Geometry check sheet. Reference: the model listing, model coordinates, mm. Face numbers are marked on the shaded views. A direction names the side the tool comes from. Give positions to 0.01 mm unless a question says otherwise; leave off trailing zeros. Order: outer loops, then holes, each group sorted by start corner. A loop starts at its lowest first (then second) coordinate and runs counter-clockwise, first axis right, second up.
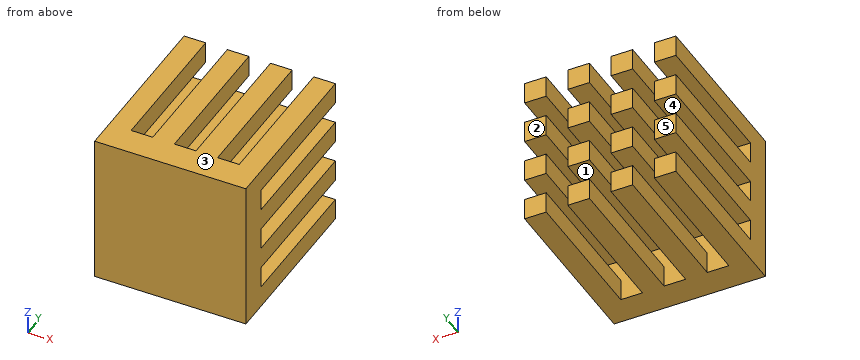
```python
from build123d import *

# Parameters (mm, degrees)
SKETCH1_W            = 10.5
SKETCH1_H            = 10.5
BOSS_EXTRUDE1_DEPTH  = 2
SKETCH2_W            = 1.5
SKETCH2_H            = 1.5
BOSS_EXTRUDE2_DEPTH  = 10
LPATTERN1_COUNT      = 4
LPATTERN1_PITCH      = 3
LPATTERN1_COUNT_DIR2 = 4
LPATTERN1_PITCH_DIR2 = 3


with BuildPart() as part:
    # Sketch1 → Boss-Extrude1 (new body)
    with BuildSketch(Plane(origin=(0, 0, 0), x_dir=(1, 0, 0), z_dir=(0, 1, 0))):
        Rectangle(SKETCH1_W, SKETCH1_H)
    extrude(amount=BOSS_EXTRUDE1_DEPTH)

    # Sketch2 → Boss-Extrude2 (add)
    with BuildSketch(Plane(origin=(0, 2, 0), x_dir=(1, 0, 0), z_dir=(0, 1, 0))):
        with Locations((-4.5, 4.5)):
            Rectangle(SKETCH2_W, SKETCH2_H)
    boss_extrude2 = extrude(amount=BOSS_EXTRUDE2_DEPTH)

    # LPattern1: Boss-Extrude2 4 × 4
    with Locations(*[(i * LPATTERN1_PITCH, 0, j * LPATTERN1_PITCH_DIR2) for i in range(LPATTERN1_COUNT) for j in range(LPATTERN1_COUNT_DIR2) if (i, j) != (0, 0)]):
        add(boss_extrude2)


solid = part.part
```
Q1. Access from +Z, -Z, +X, -X, +Y, -Y to the whole of each face (thin tool, end or side, straight path). Record for the marked faces 4 and 5.
Q2. Cross-section at B-B, the plane x = -1. Record the boundary of the cut face in (y, z).
Q3. Gauge pin test, flat end, axial feed: P1, Ø1, axis at x = 0, y = 3.5, coming from the -Z side. Record the tip position at first contact, or that the pin passes through.
Q4. Cross-section at D-D, the plane z = 0. Record the boundary of the cut face in (x, y).
Q5. Release check for a two-part mould opening along Z. For the marked faces 1, 2 and 3 record: pulls with the +Z half, pulls with the -Z half, needs draft (parallel to the pull), parting line crosses it, or undercut.
Q6. Cross-section at A-A, the plane z = -1.75. Record the boundary of the cut face in (x, y), and give its area (3 significant figures).
Q7. Thickness scan on L1, parallel to X at y = 8, z = 1.5; L2, parallel to Y at x = 1.5, z = 3. Record the ranges inside material, lowest first.
Q8. Cross-section at C-C, the plane y = 10.75. Give the number of separate pieces and of enclosed holes in the cut face, and give its area (3 significant figures).
Answers follow:
1. face 4: +X, -X, +Y
1. face 5: +Z, -Z, +X, -X, +Y
2. outline: (0, -5.25) - (12, -5.25) - (12, -3.75) - (2, -3.75) - (2, -2.25) - (12, -2.25) - (12, -0.75) - (2, -0.75) - (2, 0.75) - (12, 0.75) - (12, 2.25) - (2, 2.25) - (2, 3.75) - (12, 3.75) - (12, 5.25) - (0, 5.25) - close
3. P1: passes through
4. outline: (-5.25, 0) - (5.25, 0) - (5.25, 2) - (-5.25, 2) - close
5. face 1: undercut
5. face 2: needs draft
5. face 3: pulls with the +Z half
6. outline: (-5.25, 0) - (5.25, 0) - (5.25, 12) - (3.75, 12) - (3.75, 2) - (2.25, 2) - (2.25, 12) - (0.75, 12) - (0.75, 2) - (-0.75, 2) - (-0.75, 12) - (-2.25, 12) - (-2.25, 2) - (-3.75, 2) - (-3.75, 12) - (-5.25, 12) - close
6. area: 81.0 mm2
7. L1: x = -5.25 to -3.75, -2.25 to -0.75, 0.75 to 2.25, 3.75 to 5.25
7. L2: y = 0 to 2
8. separate pieces: 16
8. enclosed holes: 0
8. area: 36.0 mm2
